from build123d import *

# Parameters (mm, degrees)
F1_DEPTH = 10.25
F3_DEPTH = 2.25
F4_R     = 1
F5_T     = -0.9


with BuildPart() as f1:
    # F0 (on Top) → F1 (new body)
    with BuildSketch(Plane.XY):
        with BuildLine():
            Line((16, 19), (-16, 19))
            ThreePointArc((-16, 19), (-21.6568542495, 16.6568542495), (-24, 11))
            Line((-24, 11), (-24, -11))
            ThreePointArc((-24, -11), (-21.6568542495, -16.6568542495), (-16, -19))
            Line((-16, -19), (16, -19))
            ThreePointArc((16, -19), (21.6568542495, -16.6568542495), (24, -11))
            Line((24, -11), (24, 11))
            ThreePointArc((24, 11), (21.6568542495, 16.6568542495), (16, 19))
        make_face()
    extrude(amount=F1_DEPTH)

    # F2 (on face) → F3 (join)
    with BuildSketch(Plane.XY.offset(10.25)):
        with BuildLine():
            Line((12, -21.85), (12, -19))
            Line((12, -19), (-16, -19))
            ThreePointArc((-16, -19), (-21.6568542495, -16.6568542495), (-24, -11))
            Line((-24, -11), (-24, -13.85))
            ThreePointArc((-24, -13.85), (-21.6568542495, -19.5068542495), (-16, -21.85))
            Line((-16, -21.85), (12, -21.85))
        make_face()
        with BuildLine():
            Line((12, 21.85), (-16, 21.85))
            ThreePointArc((-16, 21.85), (-21.6568542495, 19.5068542495), (-24, 13.85))
            Line((-24, 13.85), (-24, 11))
            ThreePointArc((-24, 11), (-21.6568542495, 16.6568542495), (-16, 19))
            Line((-16, 19), (12, 19))
            Line((12, 19), (12, 21.85))
        make_face()
    extrude(amount=-F3_DEPTH)

    # F4
    f4_edges = [f1.edges().sort_by_distance(p)[0] for p in [
        (12, -21.85, 9.125),
        (12, 21.85, 9.125),
        (12, 19, 9.125),
        (12, -19, 9.125),
    ]]
    fillet(f4_edges, radius=F4_R)

    # F5
    f5_openings = [f1.faces().sort_by_distance(p)[0] for p in [
        (0, 0, 0),
    ]]
    offset(amount=F5_T, openings=f5_openings, kind=Kind.INTERSECTION)


solid = f1.part
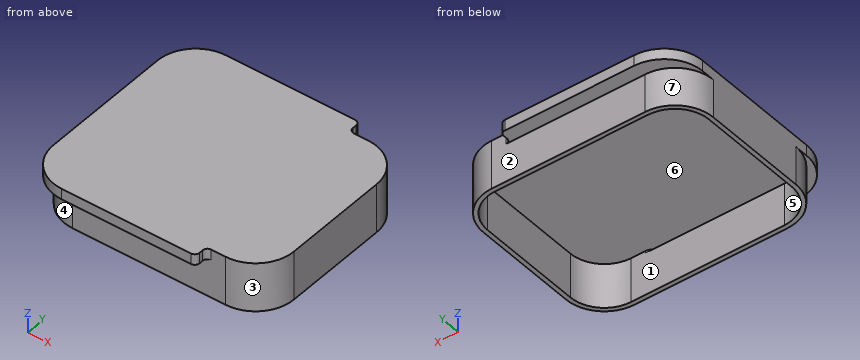
The model under review builds one solid part; all positions refer to its coordinate system, in mm. Face numbers are marked on the shaded views. A direction names the side the tool comes from. Round coordinates to 2 decimals unless told otherwise and drop trailing zeros. Write each loop counter-clockwise with the first axis right and the second up, starting at its lowest first coordinate (ties: lowest second). Pieces come first, ordered by that corner, then holes. Notation, with made-up numbers: M 56,62 L 77,62 A17 cw 77,75 Z; hole C 35,25.5 d6. An arc over 180 degrees is marked long. Answer as CSV lines item,"result". Start each with the question number.
Q1. Tool access review of the marked faces 4, 5, 6 and 7: name each direction out of +Z, -Z, +X, -X, +Y, -Y from which nothing blocks a thin tool from reaching the whole face with its end or side.
Q2. Consider section C-C, the plane x = -2. Give the boundary of the cut face in (y, z).
Q3. The part is to be moulded in two halves that separate along Y. For the marked faces 1, 2 and 3, say which applies: +Y half, -Y half, draft (parallel to the pull), parting line (faces both ways), or undercut.
Q4. Wall thickness on line 1 along Y through (x, z) = (-1, 8.5); line 2 along X through (y, z) = (-8, 2.5); line 3 along Y through (x, z) = (8, 0.5): over which ranges is each line inside the solid? List them lowest first.
Q5. Consider section D-D, the plane y = -14.5. Give the boundary of the cut face in (x, z).
Q6. Consider section A-A, the plane z = 1.5. Give the boundary of the cut face in (x, y).
Q7. Clearance check with flat-ended pins moving along their axes: P1, Ø3.5, axis at x = -6, y = -14, coming from the -Z side; P2, Ø5, axis at x = -3.5, z = 5, coming from the +Y side; P3, Ø4, axis at x = -14, z = 2, coming from the -Y side. State where each tip first meets the part, or that it passes through.
Q8. Consider section B-B, the plane y = -1.5. Give the boundary of the cut face in (x, z), then the cut area to 3 significant figures.
Result set:
1,face 4,"-Z, -X, -Y"
1,face 5,"-Z"
1,face 6,"none"
1,face 7,"-Z, -X, +Y"
2,outline,"M -21.85,8 L -19,8 L -19,0 L -18.1,0 L -18.1,8.9 L -20.95,8.9 L -20.95,9.35 L 20.95,9.35 L 20.95,8.9 L 18.1,8.9 L 18.1,0 L 19,0 L 19,8 L 21.85,8 L 21.85,10.25 L -21.85,10.25 Z"
3,face 1,"undercut"
3,face 2,"+Y half"
3,face 3,"-Y half"
4,line 1,"y = -21.85 to -18.1, 18.1 to 21.85"
4,line 2,"x = -24 to -23.1, 23.1 to 24"
4,line 3,"y = -19 to -18.1, 18.1 to 19"
5,outline,"M -23.97,8 L -23.19,8 L -23.19,0 L -22.18,0 L -22.18,8.9 L -23.07,8.9 L -23.07,9.35 L 22.18,9.35 L 22.18,0 L 23.19,0 L 23.19,10.25 L -23.97,10.25 Z"
6,outline,"M -24,-11 A8 ccw -16,-19 L 16,-19 A8 ccw 24,-11 L 24,11 A8 ccw 16,19 L -16,19 A8 ccw -24,11 Z; hole M -23.1,-11 A7.1 ccw -16,-18.1 L 16,-18.1 A7.1 ccw 23.1,-11 L 23.1,11 A7.1 ccw 16,18.1 L -16,18.1 A7.1 ccw -23.1,11 Z"
7,P1,"stops at z = 9.35"
7,P2,"stops at y = 19"
7,P3,"stops at y = -19"
8,outline,"M -24,0 L -23.1,0 L -23.1,9.35 L 23.1,9.35 L 23.1,0 L 24,0 L 24,10.25 L -24,10.25 Z"
8,area,"60.0 mm²"
